from build123d import *

# Parameters (mm, degrees)
BOSS_EXTRUDE1_DEPTH   = 12
SKETCH5_R             = 12
BOSS_EXTRUDE2_DEPTH   = 12
M6_TAPPED_HOLE1_D     = 5
BOSS_EXTRUDE3_START   = -24
BOSS_EXTRUDE3_DEPTH   = 36
BOSS_EXTRUDE3_2_DEPTH = 36
BOSS_EXTRUDE4_REACH   = 105.625
SKETCH7_W             = 18
SKETCH7_H             = 43.323398588


with BuildPart() as part:
    # Sketch1 → Boss-Extrude1 (new body)
    with BuildSketch(Plane.XY):
        with BuildLine():
            Line((-62.4, 11.757550765), (-4.8, 23.515101531))
            ThreePointArc((-4.8, 23.515101531), (-0.369908928, 23.997149151), (4.07293506, 23.65187519))
            Line((4.07293506, 23.65187519), (72.747145648, 11.825937595))
            ThreePointArc((72.747145648, 11.825937595), (82.710678119, 0), (72.747145648, -11.825937595))
            Line((72.747145648, -11.825937595), (4.07293506, -23.65187519))
            ThreePointArc((4.07293506, -23.65187519), (-0.369908928, -23.997149151), (-4.8, -23.515101531))
            Line((-4.8, -23.515101531), (-62.4, -11.757550765))
            ThreePointArc((-62.4, -11.757550765), (-72, 0), (-62.4, 11.757550765))
        make_face()
        with BuildLine():
            Line((-51.017662351, 7.957236352), (-19.153777676, 14.461424575))
            ThreePointArc((-19.153777676, 14.461424575), (-24, 0), (-19.153777676, -14.461424575))
            Line((-19.153777676, -14.461424575), (-51.017662351, -7.957236352))
            ThreePointArc((-51.017662351, -7.957236352), (-48, 0), (-51.017662351, 7.957236352))
        make_face(mode=Mode.SUBTRACT)
        with BuildLine():
            Line((18.698946243, 15.044913074), (61.487349503, 7.676601412))
            ThreePointArc((61.487349503, 7.676601412), (58.710678119, 0), (61.487349503, -7.676601412))
            Line((61.487349503, -7.676601412), (18.698946243, -15.044913074))
            ThreePointArc((18.698946243, -15.044913074), (24, 0), (18.698946243, 15.044913074))
        make_face(mode=Mode.SUBTRACT)
    extrude(amount=BOSS_EXTRUDE1_DEPTH)

    # Sketch5 → Boss-Extrude2 (add)
    with BuildSketch(Plane.XY.offset(12)):
        with Locations(Location((70.710678119, 0, 0), (0, 0, 140.229295936))):
            Circle(SKETCH5_R)
    extrude(amount=BOSS_EXTRUDE2_DEPTH)

    # M6 Tapped Hole1 (through all)
    with Locations(Plane.XY.offset(24)):
        with Locations((-60, 0), (0, 0), (70.710678119, 0)):
            Hole(M6_TAPPED_HOLE1_D / 2)

    # Boss-Extrude4: up to this face of the body (flat: up to its plane)
    boss_extrude4_end = Plane(part.part.faces().sort_by_distance((79.673131606, -7.459474336, 24))[0])
    # Sketch7 → Boss-Extrude4 (add, up to the picked face)
    with BuildSketch(Plane(origin=(0, 0, 0), x_dir=(-1, 0, 0), z_dir=(0, 0, -1)), mode=Mode.PRIVATE) as boss_extrude4_sk1:
        with Locations((-70.710678119, 29.338300706)):
            Rectangle(SKETCH7_W, SKETCH7_H)
    boss_extrude4_tool1 = split(extrude(boss_extrude4_sk1.sketch, amount=-BOSS_EXTRUDE4_REACH, mode=Mode.PRIVATE), bisect_by=boss_extrude4_end, keep=Keep.BOTH, mode=Mode.PRIVATE)


with BuildPart() as body_2:
    # Sketch6 → Boss-Extrude3 (new body)
    with BuildSketch(Plane.XY.offset(24).offset(BOSS_EXTRUDE3_START)):
        with BuildLine():
            Line((76.710678119, 24), (76.710678119, 48))
            ThreePointArc((76.710678119, 48), (79.710678119, 51), (82.710678119, 48))
            Line((82.710678119, 48), (82.710678119, 24))
            ThreePointArc((82.710678119, 24), (79.710678119, 21), (76.710678119, 24))
        make_face()
    extrude(amount=BOSS_EXTRUDE3_DEPTH)


with BuildPart() as body_3:
    # Sketch6 → Boss-Extrude3 2 (new body)
    with BuildSketch(Plane.XY.offset(24).offset(BOSS_EXTRUDE3_START)):
        with BuildLine():
            Line((58.710678119, 24), (58.710678119, 48))
            ThreePointArc((58.710678119, 48), (61.710678119, 51), (64.710678119, 48))
            Line((64.710678119, 48), (64.710678119, 24))
            ThreePointArc((64.710678119, 24), (61.710678119, 21), (58.710678119, 24))
        make_face()
    extrude(amount=BOSS_EXTRUDE3_2_DEPTH)


with BuildPart() as part_1:
    add(part.part)

    add(body_2.part)  # Boss-Extrude4 merges body 2

    add(body_3.part)  # Boss-Extrude4 merges body 3
    add(boss_extrude4_tool1.solids().sort_by(Axis((70.710678, 29.338301, 0), (0, 0, 1)))[0])


solid = part_1.part
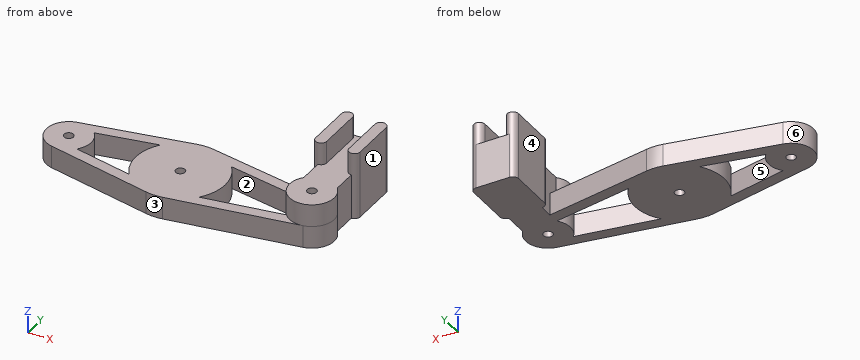
Geometry: final body of the model. Coordinates: model frame, mm. Face numbers are marked on the shaded views. A direction names the side the tool comes from. Round coordinates to 2 decimals unless told otherwise and drop trailing zeros. Loops run counter-clockwise (first coordinate to the right, second up) from the corner with the lowest first, then second, coordinate; pieces in that order, holes last. Notation, with made-up numbers: (59.25, 75) -> (91.25, 75) arc R29 ccw to (91.25, 113) -> close; hole circle Ø9 at (42, -18). An arc over 180 degrees is marked (long way). One line per question, with ' | ' between items. Start each with the question number.
1. Section C-C on x = 0. Output: boundary loops of the cut face in (y, z), and give its area (3 significant figures).
2. Set-up query: the marked faces 4, 5 and 6. Return all of +Z, -Z, +X, -X, +Y, -Y with unobstructed straight access to the full face (end or side cutting, diameter ignored); none if empty.
3. Section A-A on z = 25.5. Output: boundary loops of the cut face in (x, y).
4. Contact query for flat-ended pins moving along their axis: pin 1 (4 mm diameter, centred on x = 0, y = 0, fed in from -Z); pin 2 (4 mm diameter, centred on y = 12, z = 10, fed in from -X); pin 3 (19 mm diameter, centred on y = 36.5, z = 24, fed in from -X); pin 4 (1.5 mm diameter, centred on x = -40.5, y = -14.5, fed in from +Z). Output: stop coordinate, or through.
5. Mould query, pull axis X, two halves, no side actions, for the marked faces 1, 2 and 3. Classes: pulls with the +X half, pulls with the -X half, needs draft (parallel to the pull), parting line crosses it, or undercut.
6. Section B-B on y = 0. Output: boundary loops of the cut face in (x, z), and give its area (3 significant figures).
7. Section D-D on z = 5.5. Output: boundary loops of the cut face in (x, y).
8. Line query: line 1 along X through (y, z) = (26, 31); line 2 along Y through (x, z) = (0, 7); line 3 along Z through (x, y) = (7.5, 2). Output: solid intervals per line, ascending. Write a range as [from, to].
Returned:
1) outline: (-24, 0) -> (-2.5, 0) -> (-2.5, 12) -> (-24, 12) -> close; (2.5, 0) -> (24, 0) -> (24, 12) -> (2.5, 12) -> close | area: 516 mm2
2) face 4: +Z, -Z, -X, +Y | face 5: +Z, -Z | face 6: +Z, -Z, -X
3) outline: (58.71, 24) arc R3 ccw to (64.71, 24) -> (64.71, 48) arc R3 ccw to (58.71, 48) -> close; (76.71, 24) arc R3 ccw to (82.71, 24) -> (82.71, 48) arc R3 ccw to (76.71, 48) -> close
4) pin 1: passes through | pin 2: stops at x = -66.63 | pin 3: stops at x = 58.71 | pin 4: stops at z = 12
5) face 1: pulls with the +X half | face 2: undercut | face 3: parting line crosses it
6) outline: (-72, 0) -> (-62.5, 0) -> (-62.5, 12) -> (-72, 12) -> close; (-57.5, 0) -> (-48, 0) -> (-48, 12) -> (-57.5, 12) -> close; (-24, 0) -> (-2.5, 0) -> (-2.5, 12) -> (-24, 12) -> close; (2.5, 0) -> (24, 0) -> (24, 12) -> (2.5, 12) -> close; (58.71, 0) -> (68.21, 0) -> (68.21, 24) -> (58.71, 24) -> close; (73.21, 0) -> (82.71, 0) -> (82.71, 24) -> (73.21, 24) -> close | area: 1,200 mm2
7) outline: (-62.4, -11.76) -> (-4.8, -23.52) arc R24 ccw to (4.07, -23.65) -> (72.75, -11.83) arc R12 ccw to (79.71, 7.94) -> (79.71, 21) arc R3 ccw to (82.71, 24) -> (82.71, 48) arc R3 ccw to (79.71, 51) -> (61.71, 51) arc R3 ccw to (58.71, 48) -> (58.71, 24) arc R3 ccw to (61.71, 21) -> (61.71, 13.73) -> (4.07, 23.65) arc R24 ccw to (-4.8, 23.52) -> (-62.4, 11.76) arc R12 ccw to start; hole circle Ø5 at (-60, 0); hole (-51.02, -7.96) -> (-19.15, -14.46) arc R24 cw to (-19.15, 14.46) -> (-51.02, 7.96) arc R12 cw to start; hole circle Ø5 at (0, 0); hole (18.7, -15.04) -> (61.49, -7.68) arc R12 cw to (61.49, 7.68) -> (18.7, 15.04) arc R24 cw to start; hole circle Ø5 at (70.71, 0)
8) line 1: x = [58.71, 64.71], [76.71, 82.71] | line 2: y = [-24, -2.5], [2.5, 24] | line 3: z = [0, 12]
